Autodesk Inventor part; units mm, degrees
ref_plane "Work Plane1" through (29, 0, 0) normal (0, -1, 0) x (1, 0, 0)
ref_plane "YZ Plane" through (0, 0, 0) normal (1, 0, 0) x (0, 1, 0)
ref_plane "XZ Plane" through (0, 0, 0) normal (0, 1, 0) x (-1, 0, 0)
sketch "Szkic1" plane through (0, 0, 0) normal (0, 0, 1) x (1, 0, 0)
  line L0 (0.3333, 0) -> (14, 0)
  line L1 (14, 0) -> (14, 2)
  line L2 (14, 2) -> (2.1, 2)
  line L3 (2.1, 2) -> (1.6705, 2)
  line L4 (1.6705, 2) -> (0, 2)
  line L5 (0, 2) -> (0, 3.5)
  line L6 (0, 3.5) -> (-2.8, 3.5)
  line L7 (-2.8, 3.5) -> (-2.8, 1.4434)
  line L8 (-2.8, 1.4434) -> (-0.5, 1.4434)
  line L9 (-0.5, 1.4434) -> (0.3333, 0)
  line L10 (-6.16, 0) -> (17.36, 0)
  line L11 (0, -0.7) -> (0, 4.2)
  line L12 (2.1, 2) -> (0, 2) construction
  dimension "d1" = 11.9
  dimension "d2" = 0.4295
  dimension "d3" = 2.8
  dimension "d4" = 2.3
  dimension "d5" = 60
  dimension "d6" = 4
  dimension "d7" = 4
  dimension "d8" = 2.8868
  dimension "d9" = 7
  dimension "d26" = 14
revolve "Bryła" add sketch "Szkic1" angle 360 about axis through (0.3333, 0, 0) along (1, 0, 0) contours L9 L11 L4 L3 L2 L1 L0 | L9 L8 L7 L6 L5 L11
sketch "Szkic2" plane through (-2.8, 0, 0) normal (-1, 0, 0) x (0, 0, 1)
  circle A0 centre (0, 0) radius 1.4434
  line L0 (0, -4.9) -> (0, 4.9)
  line L1 (-4.9, 0) -> (4.9, 0)
  line L2 (1.4434, 0) -> (0.7217, -1.25)
  line L3 (0.7217, -1.25) -> (-0.7217, -1.25)
  line L4 (-0.7217, -1.25) -> (-1.4434, 0)
  line L5 (-1.4434, 0) -> (-0.7217, 1.25)
  line L6 (-0.7217, 1.25) -> (0.7217, 1.25)
  line L7 (0.7217, 1.25) -> (1.4434, 0)
  point P0 (0, 0)
extrude "Szczelina" add sketch "Szkic2" against normal up to next contours L7 A0 | A0 L2 | L6 L0 A0 | A0 L0 L3 | L0 L6 A0 | A0 L3 L0 | L4 A0 | A0 L5
fillet "Zaokrąglenie1" radius 0.4 1 edges at (-2.8, -3.5, 0)
thread "Gwint"
chamfer "Faza1" distance 0.4294 distance2 0.4294 1 edges at (14, -2, 0) measured on face at (14, 0.527, -0.2661)
ref_plane "Work Plane1" through (29, 0, 0) normal (0, -1, 0) x (1, 0, 0)
fillet "Fillet2" radius 0.1 1 edges at (0, -2, 0)
equation "\"d1\" = GEL"
equation "\"d3\" = KOH"
equation "\"d4\" = INTI"
equation "\"d6\" = GD"
equation "\"d7\" = BDM"
equation "\"d8\" = 1.1547 * SW"
equation "\"d9\" = KOD"
equation "\"d26\" = NLG"
equation "\"d30\" = R"
equation "\"d17\" = RR"
equation "\"d13\" = GEL"
equation "\"d15\" = -0.5 * SPD + 0.5 * GD"
equation "\"d16\" = GUL"
equation "\"GD\" = NND"
equation "\"NLG\" = 14"
equation "\"GEL\" = 11.9"
equation "\"KOD\" = 7"
equation "\"KOH\" = 2.8"
equation "\"INTI\" = 2.3"
equation "\"GAL\" = 0.61345 * PTC"
equation "\"GUL\" = 0.61345 * PTC"
equation "\"BDM\" = NND"
equation "\"SW\" = 2.5"
equation "\"RR\" = 0.4"
equation "\"SPD\" = NND - 1.2269 * PTC"
equation "\"R\" = 0.1"
equation "\"TOA\" = 30deg"
equation "\"GD1\" = THREADDIA - 1.2269 * PTC"
equation "\"THREADDIA\" = 4"
equation "\"FAWI\" = 45deg"
equation "\"ANG\" = 120deg"
equation "\"PTC\" = 0.7"
equation "\"NND\" = 4"
equation "\"E0\" = 1.155 * SW"
properties part number "DIN 7984 - M4 x 14" material "Stal, miękka"
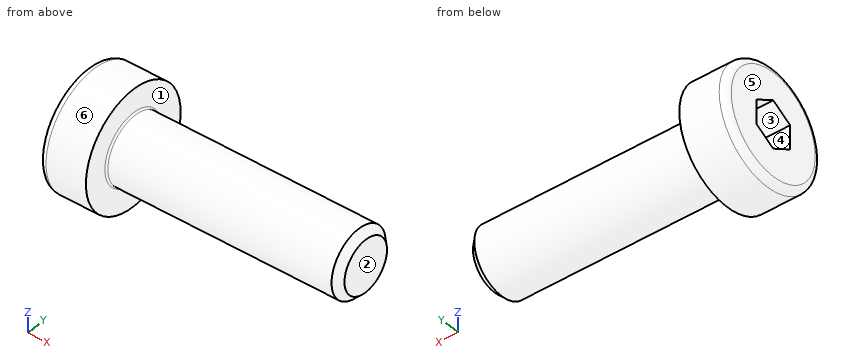
Here's how the part is built. I have some questions about the finished solid (model axes, mm). Face numbers are marked on the shaded views. A direction names the side the tool comes from. Round coordinates to 2 decimals unless told otherwise and drop trailing zeros. Loops run counter-clockwise (first coordinate to the right, second up) from the corner with the lowest first, then second, coordinate; pieces in that order, holes last.
1. Suppose I cut it at A-A, the plane x = 8.25. Please give me the cut outline in (y, z).
Answers:
outline: circle Ø4 at (0, 0)
2. Thinking about a two-plate mould opening in Z: for the marked faces 3, 4, 5 and 6, which applies, released by +Z, released by -Z, zero draft, split by the parting line, or undercut?
Answers:
face 3: undercut
face 4: undercut
face 5: zero draft
face 6: split by the parting line
3. Will these pins go through, and if not, where does the flat tip stop? pin 1 (1.5 mm diameter, centred on x = 5.5, z = 2.5, fed in from +Y); pin 2 (1 mm diameter, centred on x = -1, z = -2.5, fed in from -Y); pin 3 (4 mm diameter, centred on x = 10.5, y = 2.5, fed in from -Z).
Answers:
pin 1: stops at y = 0.97
pin 2: stops at y = -2.87
pin 3: stops at z = -1.94
4. For the marked faces 1 and 2, which set-ups out of +Z, -Z, +X, -X, +Y, -Y let a thin tool reach every point of the face, with its end or its side?
Answers:
face 1: +X
face 2: +Z, -Z, +X, +Y, -Y
5. If I drill on probe 1 along X at (y, z) = (0, 1.25); probe 2 along Y at (x, z) = (-1.5, 1); probe 3 along X at (y, z) = (-0.5, 2.5), over which ranges is the centre line in solid material (lowest first)?
Answers:
probe 1: x = -0.39 to 14
probe 2: y = -3.35 to -0.77, 0.77 to 3.35
probe 3: x = -2.8 to 0
